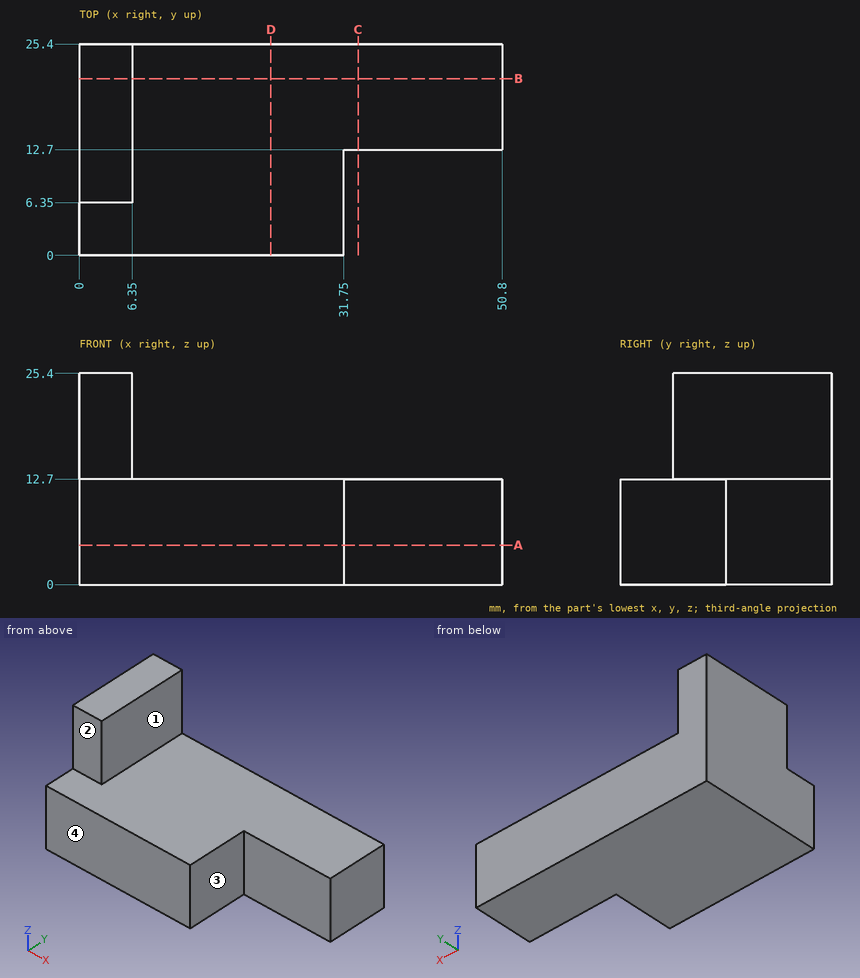
For this review, use the dimensioned drawing (mm, ordinates from the lowest corner) and the shaded views. A direction names the side the tool comes from. Round coordinates to 2 decimals unless told otherwise and drop trailing zeros. Order: outer loops, then holes, each group sorted by start corner. A loop starts at its lowest first (then second) coordinate and runs counter-clockwise, first axis right, second up. Notation, with made-up numbers: (51.25, 48) -> (79.25, 48) arc R21 ccw to (79.25, 87) -> close; hole circle Ø6 at (-17, 51). An arc over 180 degrees is marked (long way). Use CSV: the item, a comma, the result in double quotes. Start each with the question number.
(1) Consider section C-C on x = 33.5. Write out the cut boundary in (y, z).
(2) Tool access review of the marked faces 1, 2, 3 and 4: name each direction out of +Z, -Z, +X, -X, +Y, -Y from which nothing blocks a thin tool from reaching the whole face with its end or side.
(3) Consider section A-A on z = 4.75. Write out the cut boundary in (x, y), and give its area (3 significant figures).
(4) Insertion check: pin 1 (5 mm diameter, centred on x = 33.5, z = 17, fed in from +Y); pin 2 (2 mm diameter, centred on y = 10.5, z = 22.5, fed in from +X); pin 3 (6.5 mm diameter, centred on x = 42.5, z = 6.5, fed in from -Y); pin 4 (5 mm diameter, centred on y = 8.5, z = 14, fed in from +X). Each pin has a flat end and moves straight along its axis. Give the tip position at first contact, or say it passes through.
(5) Consider section B-B on y = 21.25. Write out the cut boundary in (x, z), and give its area (3 significant figures).
(6) Wall thickness on probe 1 along Y at (x, z) = (43.5, 8.25); probe 2 along X at (y, z) = (23, 19.5); probe 3 along X at (y, z) = (10.25, 4.5): over which ranges is each line inside the solid? List them lowest first. Write a range as from..to.
(7) Consider section D-D on x = 23. Write out the cut boundary in (y, z).
Responses:
1,outline,"(12.7, 0) -> (25.4, 0) -> (25.4, 12.7) -> (12.7, 12.7) -> close"
2,face 1,"+Z, +X, +Y, -Y"
2,face 2,"+Z, +X, -X, -Y"
2,face 3,"+Z, -Z, +X, -Y"
2,face 4,"+Z, -Z, +X, -X, -Y"
3,outline,"(0, 0) -> (31.75, 0) -> (31.75, 12.7) -> (50.8, 12.7) -> (50.8, 25.4) -> (0, 25.4) -> close"
3,area,"1,050 mm²"
4,pin 1,"through"
4,pin 2,"x = 6.35"
4,pin 3,"y = 12.7"
4,pin 4,"x = 31.75"
5,outline,"(0, 0) -> (50.8, 0) -> (50.8, 12.7) -> (6.35, 12.7) -> (6.35, 25.4) -> (0, 25.4) -> close"
5,area,"726 mm²"
6,probe 1,"12.7..25.4"
6,probe 2,"0..6.35"
6,probe 3,"0..31.75"
7,outline,"(0, 0) -> (25.4, 0) -> (25.4, 12.7) -> (0, 12.7) -> close"
